Check sheet for the modelled part. Datum: model origin and axes. Units: mm. A direction names the side the tool comes from. Coordinates: 2 decimals unless noted, no trailing zeros. Loops run counter-clockwise (first coordinate to the right, second up) from the corner with the lowest first, then second, coordinate; pieces in that order, holes last. Notation, with made-up numbers: (26.5, 72.5) - (53.5, 72.5) arc R28 ccw to (53.5, 98.5) - close; hole circle Ø8 at (80, -12). An arc over 180 degrees is marked (long way). Answer as a JSON object with one key per item and string values. Group by question number.
from build123d import *

# Parameters (mm, degrees)
SKETCH_W        = 34
SKETCH_H        = 34
PAD_DEPTH       = 80
POCKET_DEPTH    = 80
SKETCH002_R     = 3
POCKET001_DEPTH = 4
SKETCH003_R     = 3
POCKET002_DEPTH = 4
SKETCH004_R     = 4
POCKET003_DEPTH = 2
SKETCH005_R     = 4
POCKET004_DEPTH = 2
SKETCH006_W     = 6.4
SKETCH006_H     = 2
SKETCH006_H_2   = 7
POCKET005_DEPTH = 12
SKETCH007_W     = 6.4
SKETCH007_H     = 2
SKETCH007_W_2   = 6
SKETCH007_H_2   = 6.6
POCKET006_DEPTH = 12
CHAMFER_SIZE    = 1.98
SKETCH008_W     = 8
SKETCH008_H     = 5
POCKET007_DEPTH = 80
SKETCH009_W     = 9.188405
SKETCH009_H     = 3.137501
POCKET008_DEPTH = 8
SKETCH010_W     = 8.306599
SKETCH010_H     = 2.918531
POCKET009_DEPTH = 8


with BuildPart() as part:
    # Sketch → Pad (new body)
    with BuildSketch(Plane.XY):
        with Locations((17, 17)):
            Rectangle(SKETCH_W, SKETCH_H)
    extrude(amount=PAD_DEPTH)

    # Sketch001 (on Face6 of Pad) → Pocket (cut)
    with BuildSketch(Plane.XY.offset(80)):
        Polygon((6.5, 27.5), (14, 27.5), (14, 23.5), (17, 21), (20, 23.5), (20, 27.5), (27.5, 27.5), (27.5, 19.5), (23.5, 19.5), (21, 17), (23.5, 14), (27.5, 14), (27.5, 6.5), (20, 6.5), (20, 10.5), (17, 13), (14, 10.5), (14, 6.5), (6.5, 6.5), (6.5, 14), (10.5, 14), (13, 17), (10.5, 19.5), (6.5, 19.5), align=None)
    extrude(amount=-POCKET_DEPTH, mode=Mode.SUBTRACT)

    # Sketch002 (on Face2 of Pocket) → Pocket001 (cut)
    with BuildSketch(Plane(origin=(0, 0, 0), x_dir=(0, -1, 0), z_dir=(-1, 0, 0))):
        with Locations((-17, 60)):
            Circle(SKETCH002_R)
        with Locations((-17, 20)):
            Circle(SKETCH002_R)
    extrude(amount=-POCKET001_DEPTH, mode=Mode.SUBTRACT)

    # Sketch003 (on Face3 of Pocket001) → Pocket002 (cut)
    with BuildSketch(Plane.YZ.offset(34)):
        with Locations((17, 60)):
            Circle(SKETCH003_R)
        with Locations((17, 20)):
            Circle(SKETCH003_R)
    extrude(amount=-POCKET002_DEPTH, mode=Mode.SUBTRACT)

    # Sketch004 (on Face1 of Pocket002) → Pocket003 (cut)
    with BuildSketch(Plane(origin=(0, 34, 0), x_dir=(-1, 0, 0), z_dir=(0, 1, 0))):
        with Locations((-27, 60)):
            Circle(SKETCH004_R)
        with Locations((-7, 60)):
            Circle(SKETCH004_R)
        with Locations((-27, 20)):
            Circle(SKETCH004_R)
        with Locations((-7, 20)):
            Circle(SKETCH004_R)
    extrude(amount=-POCKET003_DEPTH, mode=Mode.SUBTRACT)

    # Sketch005 (on Face10 of Pocket003) → Pocket004 (cut)
    with BuildSketch(Plane.XZ):
        with Locations((7, 60)):
            Circle(SKETCH005_R)
        with Locations((27, 60)):
            Circle(SKETCH005_R)
        with Locations((7, 20)):
            Circle(SKETCH005_R)
        with Locations((27, 20)):
            Circle(SKETCH005_R)
    extrude(amount=-POCKET004_DEPTH, mode=Mode.SUBTRACT)

    # Sketch006 (on Face4 of Pocket004) → Pocket005 (cut)
    with BuildSketch(Plane.XY.offset(80)):
        with Locations((17, 1)):
            Rectangle(SKETCH006_W, SKETCH006_H)
        with Locations((17, 10)):
            Rectangle(SKETCH006_W, SKETCH006_H_2)
    extrude(amount=-POCKET005_DEPTH, mode=Mode.SUBTRACT)

    # Sketch007 (on Face3 of Pocket005) → Pocket006 (cut)
    with BuildSketch(Plane(origin=(0, 0, 0), x_dir=(1, 0, 0), z_dir=(0, 0, -1))):
        with Locations((17, -1)):
            Rectangle(SKETCH007_W, SKETCH007_H)
        with Locations((17, -9.8)):
            Rectangle(SKETCH007_W_2, SKETCH007_H_2)
    extrude(amount=-POCKET006_DEPTH, mode=Mode.SUBTRACT)

    # Chamfer
    chamfer_edges = [part.edges().sort_by_distance(p)[0] for p in [
        (17, 21, 40),
    ]]
    chamfer(chamfer_edges, length=CHAMFER_SIZE)

    # Sketch008 (on Face1 of Chamfer) → Pocket007 (cut)
    with BuildSketch(Plane(origin=(0, 0, 0), x_dir=(1, 0, 0), z_dir=(0, 0, -1))):
        with Locations((17, -24.5)):
            Rectangle(SKETCH008_W, SKETCH008_H)
    extrude(amount=-POCKET007_DEPTH, mode=Mode.SUBTRACT)

    # Sketch009 (on Face8 of Pocket007) → Pocket008 (cut)
    with BuildSketch(Plane.XZ.offset(-2)):
        with Locations((17.216907, 69.686737)):
            Rectangle(SKETCH009_W, SKETCH009_H)
    extrude(amount=-POCKET008_DEPTH, mode=Mode.SUBTRACT)

    # Sketch010 (on Face8 of Pocket008) → Pocket009 (cut)
    with BuildSketch(Plane.XZ.offset(-2)):
        with Locations((16.61403, 10.454884)):
            Rectangle(SKETCH010_W, SKETCH010_H)
    extrude(amount=-POCKET009_DEPTH, mode=Mode.SUBTRACT)


solid = part.part
1. Material ranges on line 1 (Z direction, x = 7, y = 0.4); line 2 (Z direction, x = 2.05, y = 17); line 3 (X direction, y = 9.5, z = 62), recorded low to high.
2. Release check for a two-part mould opening along Y. For faces 1 (the face through (27, 2, 60)), 2 (the face through (30, 17, 60)), 3 (the face through (15.521, 11.768, 40.392)), 4 (the face through (29.95, 33.01, 22.7)) record: released by +Y, released by -Y, zero draft, split by the parting line, or undercut.
3. Sectioned sample at B-B on y = 16. Record the cut outline in (x, z).
4. Gauge pin test, flat ends, axial feed: pin 1 (5 mm diameter, centred on x = 26.5, z = 19.5, fed in from -Y); pin 2 (7 mm diameter, centred on x = 7, z = 60, fed in from +Y); pin 3 (5 mm diameter, centred on x = 16.5, y = 9.5, fed in from +Z). Record the tip position at first contact, or that the pin passes through.
5. Sectioned sample at A-A on z = 27.5. Record the cut outline in (x, y), plus the area to 3 significant figures.
6. Access from +Z, -Z, +X, -X, +Y, -Y to the whole of each face (thin tool, end or side, straight path). Record for faces 5 (the face through (12.461, 4, 10)), 6 (the face through (26, 19.5, 41)), 7 (the face through (17, 9, 68)).
Answers follow:
{
 "1": {"line 1": "z = 0 to 16, 24 to 56, 64 to 80", "line 2": "z = 0 to 17, 23 to 57, 63 to 80", "line 3": "x = 0 to 6.5, 14 to 20, 27.5 to 34"},
 "2": {"face 1": "released by -Y", "face 2": "undercut", "face 3": "undercut", "face 4": "zero draft"},
 "3": {"outline": "(0, 0) - (12.17, 0) - (12.17, 80) - (0, 80) - (0, 62.83) - (4, 62.83) - (4, 57.17) - (0, 57.17) - (0, 22.83) - (4, 22.83) - (4, 17.17) - (0, 17.17) - close; (21.83, 0) - (34, 0) - (34, 17.17) - (30, 17.17) - (30, 22.83) - (34, 22.83) - (34, 57.17) - (30, 57.17) - (30, 62.83) - (34, 62.83) - (34, 80) - (21.83, 80) - close"},
 "4": {"pin 1": "stops at y = 2", "pin 2": "stops at y = 32", "pin 3": "stops at z = 68"},
 "5": {"outline": "(0, 0) - (34, 0) - (34, 34) - (0, 34) - close; hole (6.5, 6.5) - (14, 6.5) - (14, 10.5) - (17, 13) - (20, 10.5) - (20, 6.5) - (27.5, 6.5) - (27.5, 14) - (23.5, 14) - (21, 17) - (23.5, 19.5) - (27.5, 19.5) - (27.5, 27.5) - (20, 27.5) - (20, 27) - (14, 27) - (14, 27.5) - (6.5, 27.5) - (6.5, 19.5) - (10.5, 19.5) - (13, 17) - (10.5, 14) - (6.5, 14) - close", "area": "807 mm^2"},
 "6": {"face 5": "none", "face 6": "+Z, -Z", "face 7": "+Z"}
}
